from build123d import *

# Parameters (mm, degrees)
F1_DEPTH = 2083.59375
F3_DEPTH = 115.8885
F5_DEPTH = 949.325
F6_W     = 6.35
F6_H     = 30.1625
F7_DEPTH = 2083.59475


with BuildPart() as f1:
    # F0 (on Top) → F1 (new body)
    with BuildSketch(Plane.XY):
        Polygon((0, 73.025), (0, 115.8875), (-17.4625, 115.8875), (-17.4625, 79.375), (-26.9875, 79.375), (-26.9875, 36.5125), (-17.4625, 36.5125), (-17.4625, 0), (0, 0), (0, 42.8625), (-6.35, 42.8625), (-6.35, 73.025), align=None)
        Polygon((-949.325, 115.8875), (-949.325, 73.025), (-942.975, 73.025), (-942.975, 42.8625), (-949.325, 42.8625), (-949.325, 0), (-931.8625, 0), (-931.8625, 36.5125), (-922.3375, 36.5125), (-922.3375, 79.375), (-931.8625, 79.375), (-931.8625, 115.8875), align=None)
    extrude(amount=F1_DEPTH)

    # F2 (on Front) → F3 (cut, through all)
    with BuildSketch(Plane.XZ):
        Polygon((0, 2083.59375), (-949.325, 2083.59375), (-474.6625, 1608.93125), align=None)
    extrude(amount=-F3_DEPTH, mode=Mode.SUBTRACT)

    # F4 (on Right) → F5 (join, through all)
    with BuildSketch(Plane.YZ):
        Polygon((79.375, 2066.13125), (115.8875, 2066.13125), (115.8875, 2083.59375), (73.025, 2083.59375), (73.025, 2077.24375), (42.8625, 2077.24375), (42.8625, 2083.59375), (0, 2083.59375), (0, 2066.13125), (36.5125, 2066.13125), (36.5125, 2056.60625), (79.375, 2056.60625), align=None)
    extrude(amount=-F5_DEPTH)

    # F6 (on Top) → F7 (cut, through all)
    with BuildSketch(Plane.XY):
        with Locations((-3.175, 57.94375)):
            Rectangle(F6_W, F6_H)
        with Locations((-946.15, 57.94375)):
            Rectangle(F6_W, F6_H)
    extrude(amount=F7_DEPTH, mode=Mode.SUBTRACT)


solid = f1.part
Read the model definition and answer for the solid it produces. Units are mm, in the model's axes. A direction names the side the tool comes from. Round coordinates to 2 decimals unless told otherwise and drop trailing zeros. Loops run counter-clockwise (first coordinate to the right, second up) from the corner with the lowest first, then second, coordinate; pieces in that order, holes last.
Q1. Determine the mould class of faces 5 (the face through (-15, 115.888, 1037)), 6 (the face through (0, 94, 1027)), 7 (the face through (-931.862, 97, 1019)) for opening direction X: released by +X, released by -X, zero draft, split by the parting line, or undercut.
Q2. Each of these flat-tipped pins is pushed along its axis until it touches: pin 1 (15 mm diameter, centred on y = 56.5, z = 638.5, fed in from -X) (3 decimals); pin 2 (21.5 mm diameter, centred on x = -663.5, y = 58, fed in from -Z); pin 3 (13 mm diameter, centred on y = 61, z = 600, fed in from +X). Where does it stop, or does it pass through?
Q3. Which of the six approach directions +Z, -Z, +X, -X, +Y, -Y give full straight-line access (tool end or side, diameter ignored) to faces 1 (the face through (-468, 58, 2056.606)), 2 (the face through (-931.862, 18, 1019)), 3 (the face through (-17.462, 98, 1019)), 4 (the face through (-934, 0, 1037))?
Q4. Consider probe 1 along X at (y, z) = (40, 1285) (1 decimal); probe 2 along X at (y, z) = (92.5, 1819) (1 decimal); probe 3 along Z at (x, y) = (-621, 106). Determine where each line is inside the solid, lowest interval first.
Q5. Section B-B on x = -567.5 is taken. Write down the section's boundary in (y, z) (1 decimal).
Output:
1. face 5: zero draft
1. face 6: released by +X
1. face 7: undercut
2. pin 1: stops at x = -942.975
2. pin 2: stops at z = 2056.61
2. pin 3: stops at x = -6.35
3. face 1: -Z, +Y, -Y
3. face 2: -Z, -Y
3. face 3: -Z, +Y
3. face 4: +Z, -Z, +X, -X, -Y
4. probe 1: x = -949.3 to -922.3, -27 to 0
4. probe 2: x = -949.3 to -931.9, -17.5 to 0
4. probe 3: z = 2066.13 to 2083.59
5. outline: (0, 2066.1) - (36.5, 2066.1) - (36.5, 2056.6) - (79.4, 2056.6) - (79.4, 2066.1) - (115.9, 2066.1) - (115.9, 2083.6) - (73, 2083.6) - (73, 2077.2) - (42.9, 2077.2) - (42.9, 2083.6) - (0, 2083.6) - close
